from build123d import *

# Parameters (mm, degrees)
SKETCH_W        = 28.575
SKETCH_H        = 44.45
PAD_DEPTH       = 15.875
SKETCH002_W     = 19.558
SKETCH002_H     = 19.558
POCKET_DEPTH    = 15.876
SKETCH003_W     = 15.875
SKETCH003_H     = 12.7
POCKET001_DEPTH = 12.7
SKETCH004_R     = 3.9878
POCKET002_DEPTH = 28.576
SKETCH005_R     = 1.5875
POCKET003_DEPTH = 44.451
POCKET004_DEPTH = 3.2


with BuildPart() as part:
    # Sketch → Pad (new body)
    with BuildSketch(Plane.XY):
        with Locations((14.2875, 22.225)):
            Rectangle(SKETCH_W, SKETCH_H)
    extrude(amount=PAD_DEPTH)

    # Sketch002 → Pocket (cut, through all)
    with BuildSketch(Plane(origin=(0, 0, 0), x_dir=(1, 0, 0), z_dir=(0, 0, -1))):
        with Locations((14.2875, -30.1625)):
            Rectangle(SKETCH002_W, SKETCH002_H)
    extrude(amount=-POCKET_DEPTH, mode=Mode.SUBTRACT)

    # Sketch003 → Pocket001 (cut)
    with BuildSketch(Plane.XY.offset(15.875)):
        with Locations((14.2875, 6.35)):
            Rectangle(SKETCH003_W, SKETCH003_H)
    extrude(amount=-POCKET001_DEPTH, mode=Mode.SUBTRACT)

    # Sketch004 → Pocket002 (cut, through all)
    with BuildSketch(Plane.YZ.offset(28.575)):
        with Locations((6.35, 9.525)):
            Circle(SKETCH004_R)
        with BuildLine():
            ThreePointArc((6.35, 15.875), (1.859872, 14.015128), (0, 9.525))
            Line((0, 9.525), (0, 15.875))
            Line((0, 15.875), (6.35, 15.875))
        make_face()
    extrude(amount=-POCKET002_DEPTH, mode=Mode.SUBTRACT)

    # Sketch005 → Pocket003 (cut, through all)
    with BuildSketch(Plane(origin=(0, 44.45, 0), x_dir=(-1, 0, 0), z_dir=(0, 1, 0))):
        with Locations((-14.2875, 7.9375)):
            Circle(SKETCH005_R)
    extrude(amount=-POCKET003_DEPTH, mode=Mode.SUBTRACT)

    # Sketch006 → Pocket004 (cut)
    with BuildSketch(Plane(origin=(0, 20.3835, 0), x_dir=(-1, 0, 0), z_dir=(0, 1, 0))):
        Polygon((-16.287496, 11.401586), (-12.287504, 11.401586), (-10.287508, 7.937492), (-12.287504, 4.473397), (-16.287496, 4.473397), (-18.287492, 7.937492), align=None)
    extrude(amount=-POCKET004_DEPTH, mode=Mode.SUBTRACT)


solid = part.part
CAD build for the part. Positions are in the model's coordinates, mm. A direction names the side the tool comes from. Coordinates: 2 decimals unless noted, no trailing zeros. Order: outer loops, then holes, each group sorted by start corner. A loop starts at its lowest first (then second) coordinate and runs counter-clockwise, first axis right, second up.
Item 1: Band-saw the part on C-C on y = 4. List the corners of the cut face in (x, z) (3 decimals).
Check sheet entries:
outline: (0, 0) - (28.575, 0) - (28.575, 6.303) - (22.225, 6.303) - (22.225, 3.175) - (6.35, 3.175) - (6.35, 6.303) - (0, 6.303) - close; (0, 12.747) - (6.35, 12.747) - (6.35, 15.424) - (0, 15.424) - close; (22.225, 12.747) - (28.575, 12.747) - (28.575, 15.424) - (22.225, 15.424) - close
Item 2: Pin check, flat tips, straight feed: pin 1 Ø1 at (x, y) = (14.5, 38.5) entering from +Z; pin 2 Ø4 at (x, z) = (13.5, 7.5) entering from -Y; pin 3 Ø6.5 at (x, y) = (12, 4.5) entering from +Z (3 decimals). Stop position of each tip, or through.
Check sheet entries:
pin 1: passes through
pin 2: stops at y = 12.7
pin 3: stops at z = 3.175
Item 3: Two-plate mould, pull along Y, no slides. Class faces 5 (the face through (0, 22, 8)), 6 (the face through (14, 19, 4.473)), 7 (the face through (14, 44.45, 6)), 8 (the face through (14, 19, 11.402)): +Y half, -Y half, draft (parallel to the pull), parting line (faces both ways), or undercut.
Check sheet entries:
face 5: draft
face 6: undercut
face 7: +Y half
face 8: undercut
Item 4: Drill centre lines: L1, parallel to X at y = 4.5, z = 5.75 (3 decimals); L2, parallel to Z at x = 24, y = 6.35 (3 decimals); L3, parallel to Y at x = 20.5, z = 9.5. Where is each one in solid material? Low to high.
Check sheet entries:
L1: x = 0 to 6.35, 22.225 to 28.575
L2: z = 0 to 5.537, 13.513 to 15.875
L3: y = 12.7 to 20.38, 39.94 to 44.45
Item 5: 3-axis set-ups, long thin cutter, end or side, ignore diameter. For faces 1 (the face through (11.274, 18.806, 6.23)), 2 (the face through (14, 39.942, 6)), 3 (the face through (14, 0, 3)), 4 (the face through (22.225, 6, 5)): which of +Z, -Z, +X, -X, +Y, -Y reach the whole face in a straight line?
Check sheet entries:
face 1: none
face 2: +Z, -Z
face 3: +Z, -Z, +X, -X, -Y
face 4: +Z, -Y
Item 6: Band-saw the part on A-A on y = 21. List the corners of the cut face in (x, z) (1 decimal), plus the area to 3 significant figures.
Check sheet entries:
outline: (0, 0) - (4.5, 0) - (4.5, 15.9) - (0, 15.9) - close; (24.1, 0) - (28.6, 0) - (28.6, 15.9) - (24.1, 15.9) - close
area: 143 mm2
